from build123d import *

# Parameters (mm, degrees)
F2_R      = 70
F2_R_2    = 59.5
F3_DEPTH  = 20
F4_R      = 15
F5_DEPTH  = 5
F6_W      = 130
F6_H      = 15
F7_DEPTH  = 5
F8_W      = 15
F8_H      = 130
F9_DEPTH  = 5
F11_R     = 3
F12_DEPTH = 5.001
F14_DEPTH = 25


with BuildPart() as f3:
    # F2 (on Front) → F3 (new body)
    with BuildSketch(Plane.XZ):
        Circle(F2_R)
        Circle(F2_R_2, mode=Mode.SUBTRACT)
    extrude(amount=F3_DEPTH)


with BuildPart() as f5:
    # F4 (on Front) → F5 (new body)
    with BuildSketch(Plane.XZ):
        Circle(F4_R)
    extrude(amount=F5_DEPTH)


with BuildPart() as f7:
    # F6 (on Front) → F7 (new body)
    with BuildSketch(Plane.XZ):
        Rectangle(F6_W, F6_H)
    extrude(amount=F7_DEPTH)


with BuildPart() as f9:
    # F8 (on Front) → F9 (new body)
    with BuildSketch(Plane.XZ):
        Rectangle(F8_W, F8_H)
    extrude(amount=F9_DEPTH)


with BuildPart() as f3_1:
    add(f3.part)

    # F10: union F5, F7, F9
    add(f5.part)
    add(f7.part)
    add(f9.part)

    # F11 (on face) → F12 (cut, through all)
    with BuildSketch(Plane.XZ.offset(5)):
        Circle(F11_R)
    extrude(amount=-F12_DEPTH, mode=Mode.SUBTRACT)

    # F13 (on Front) → F14 (cut)
    with BuildSketch(Plane.XZ):
        with BuildLine():
            ThreePointArc((0.65, -11.5), (0.4596194078, -11.0403805922), (0, -10.85))
            ThreePointArc((0, -10.85), (-0.4596194078, -11.9596194078), (0.65, -11.5))
        make_face()
        with BuildLine():
            ThreePointArc((0.65, 11.5), (-0.4596194078, 11.9596194078), (0, 10.85))
            ThreePointArc((0, 10.85), (0.4596194078, 11.0403805922), (0.65, 11.5))
        make_face()
    extrude(amount=F14_DEPTH, mode=Mode.SUBTRACT)


solid = f3_1.part
The model under review builds one solid part; all positions refer to its coordinate system, in mm. A direction names the side the tool comes from. Round coordinates to 2 decimals unless told otherwise and drop trailing zeros. Loops run counter-clockwise (first coordinate to the right, second up) from the corner with the lowest first, then second, coordinate; pieces in that order, holes last. Notation, with made-up numbers: (21, 56.25) -> (67, 56.25) arc R19 ccw to (67, 81.25) -> close; hole circle Ø8 at (28.5, 17.25). An arc over 180 degrees is marked (long way). One line per question, with ' | ' between items. Start each with the question number.
Item 1: Machinability: for faces 4 (the face through (0, -5, 5)), 5 (the face through (-31, -20, -52)), 6 (the face through (-7.5, -2, 36)), which of the approach directions +Z, -Z, +X, -X, +Y, -Y give a long, thin tool a straight path to every point of the face, cutting with its end or side? Answer none if there is none.
Item 2: For pin 1 (1.5 mm diameter, centred on x = 43.5, y = -2.5, fed in from +Z); pin 2 (2 mm diameter, centred on y = -14.5, z = 9.5, fed in from +X); pin 3 (1.5 mm diameter, centred on y = -1.5, z = -37, fed in from +X); pin 4 (2 mm diameter, centred on x = 0, z = 11.5, fed in from +Y), all flat-tipped, find the tip position at first contact; note any pin that passes through.
Item 3: Wall thickness on line 1 along Z through (x, y) = (0, -9); line 2 along X through (y, z) = (-4.75, 49.5); line 3 along X through (y, z) = (-3.05, 11.5): over which ranges is each line inside the solid? List them lowest first. Write a range as [from, to].
Item 4: Add section D-D, the plane y = -12.25. Write out the cut boundary in (x, z).
Item 5: Draft analysis for pull direction X (two halves, no side actions). For faces 1 (the face through (-55.55, -9.86, -42.594)), 2 (the face through (7.5, -2, 36)), 3 (the face through (-1, 0, -15)), state which applies: +X half, -X half, draft (parallel to the pull), parting line (faces both ways), or undercut.
Item 6: Add section A-A, the plane z = 0. Write out the cut boundary in (x, y).
Item 7: Add section B-B, the plane x = -45. Write out the cut boundary in (y, z), then the cut area to 3 significant figures.
Item 8: Add section C-C, the plane z = -25.5. Write out the cut boundary in (x, y), then the cut area to 3 significant figures.
Return value:
1) face 4: -Y | face 5: +Z, -Z, +X, -X, -Y | face 6: +Y, -Y
2) pin 1: stops at z = 55.43 | pin 2: stops at x = 69.48 | pin 3: stops at x = 59.88 | pin 4: stops at y = 0
3) line 1: z = [-70, -59.5], [59.5, 70] | line 2: x = [-49.49, -33.02], [-7.5, 7.5], [33.02, 49.49] | line 3: x = [-69.05, -58.38], [-9.63, -0.65], [0.65, 9.63], [58.38, 69.05]
4) outline: circle Ø140 at (0, 0); hole circle Ø119 at (0, 0)
5) face 1: parting line | face 2: undercut | face 3: draft
6) outline: (-70, -20) -> (-59.5, -20) -> (-59.5, -5) -> (-3, -5) -> (-3, 0) -> (-70, 0) -> close; (3, -5) -> (59.5, -5) -> (59.5, -20) -> (70, -20) -> (70, 0) -> (3, 0) -> close
7) outline: (-20, -53.62) -> (0, -53.62) -> (0, -38.93) -> (-20, -38.93) -> close; (-20, 38.93) -> (0, 38.93) -> (0, 53.62) -> (-20, 53.62) -> close; (-5, -7.5) -> (0, -7.5) -> (0, 7.5) -> (-5, 7.5) -> close | area: 663 mm2
8) outline: (-65.19, -20) -> (-53.76, -20) -> (-53.76, 0) -> (-65.19, 0) -> close; (-7.5, -5) -> (7.5, -5) -> (7.5, 0) -> (-7.5, 0) -> close; (53.76, -20) -> (65.19, -20) -> (65.19, 0) -> (53.76, 0) -> close | area: 532 mm2
